Study the drawing (mm; zero at the part's minimum x, y, z) and answer. A direction names the side the tool comes from. Round coordinates to 2 decimals unless told otherwise and drop trailing zeros. Write each loop counter-clockwise with the first axis right and the second up, starting at its lowest first coordinate (ties: lowest second). Pieces come first, ordered by that corner, then holes. Notation, with made-up numbers: (18, 30.5) -> (77, 30.5) arc R20 cw to (77, 63.5) -> close; hole circle Ø10 at (-12.75, 28.5). An arc over 180 degrees is marked (long way). Return JSON: item names as keys, results as strings.
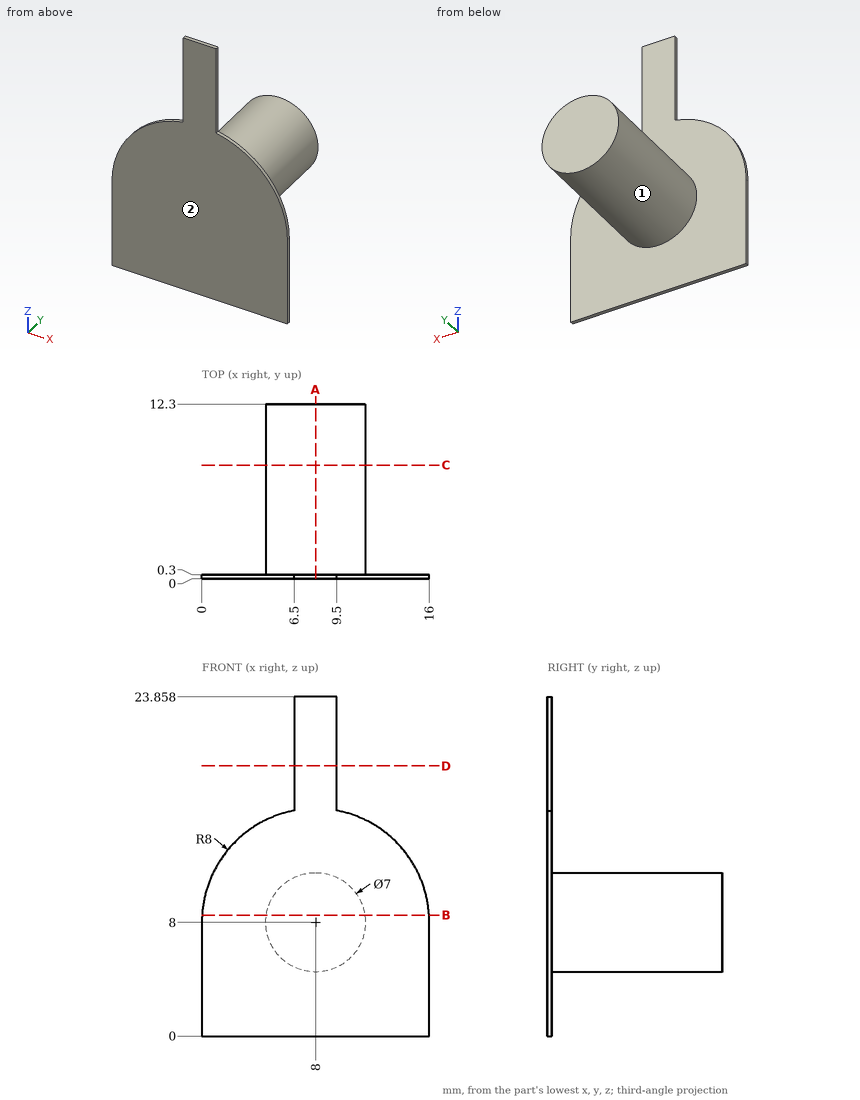
Item 1: Section A-A (x = 8) is taken. Give the vertices of the cut face in (y, z).
Worked answers:
{"outline": "(0, 0) -> (0.3, 0) -> (0.3, 4.5) -> (12.3, 4.5) -> (12.3, 11.5) -> (0.3, 11.5) -> (0.3, 23.86) -> (0, 23.86) -> close"}
Item 2: Flat-ended cylindrical pins translate along their axes: pin 1 (3 mm diameter, centred on x = 4.5, y = 1.5, fed in from +Z); pin 2 (1.5 mm diameter, centred on x = 9.5, y = 8, fed in from +Z); pin 3 (4 mm diameter, centred on x = 11, y = 7.5, fed in from -Z). Find the tip coordinate at first contact, or state that the pin passes through.
Worked answers:
{"pin 1": "stops at z = 15.57", "pin 2": "stops at z = 11.42", "pin 3": "stops at z = 4.65"}
Item 3: Section C-C (y = 8) is taken. Give the vertices of the cut face in (x, z), then the cut area to 3 significant figures.
Worked answers:
{"outline": "circle Ø7 at (8, 8)", "area": "38.5 mm2"}
Item 4: A tool of negligible diameter and unlimited length cuts with its end or side. For the marked faces 1 and 2, from which of +Z, -Z, +X, -X, +Y, -Y can it reach the whole face along a straight path? Write none if from no direction.
Worked answers:
{"face 1": "+Y", "face 2": "+Z, -Z, +X, -X, -Y"}
Item 5: Section D-D (z = 19) is taken. Give the vertices of the cut face in (x, y).
Worked answers:
{"outline": "(6.5, 0) -> (9.5, 0) -> (9.5, 0.3) -> (6.5, 0.3) -> close"}
Item 6: Straight lines are drawn through the part: L1, parallel to Y at x = 11, z = 10.5; L2, parallel to Z at x = 10, y = 1.25; L3, parallel to Z at x = 5.5, y = 11. For each, find the intervals that lie inside material, in ascending order. Write a range as [from, to].
Worked answers:
{"L1": "y = [0, 0.3]", "L2": "z = [5.13, 10.87]", "L3": "z = [5.55, 10.45]"}
Item 7: Section B-B (z = 8.5) is taken. Give the vertices of the cut face in (x, y).
Worked answers:
{"outline": "(0.02, 0) -> (15.98, 0) -> (15.98, 0.3) -> (11.46, 0.3) -> (11.46, 12.3) -> (4.54, 12.3) -> (4.54, 0.3) -> (0.02, 0.3) -> close"}
